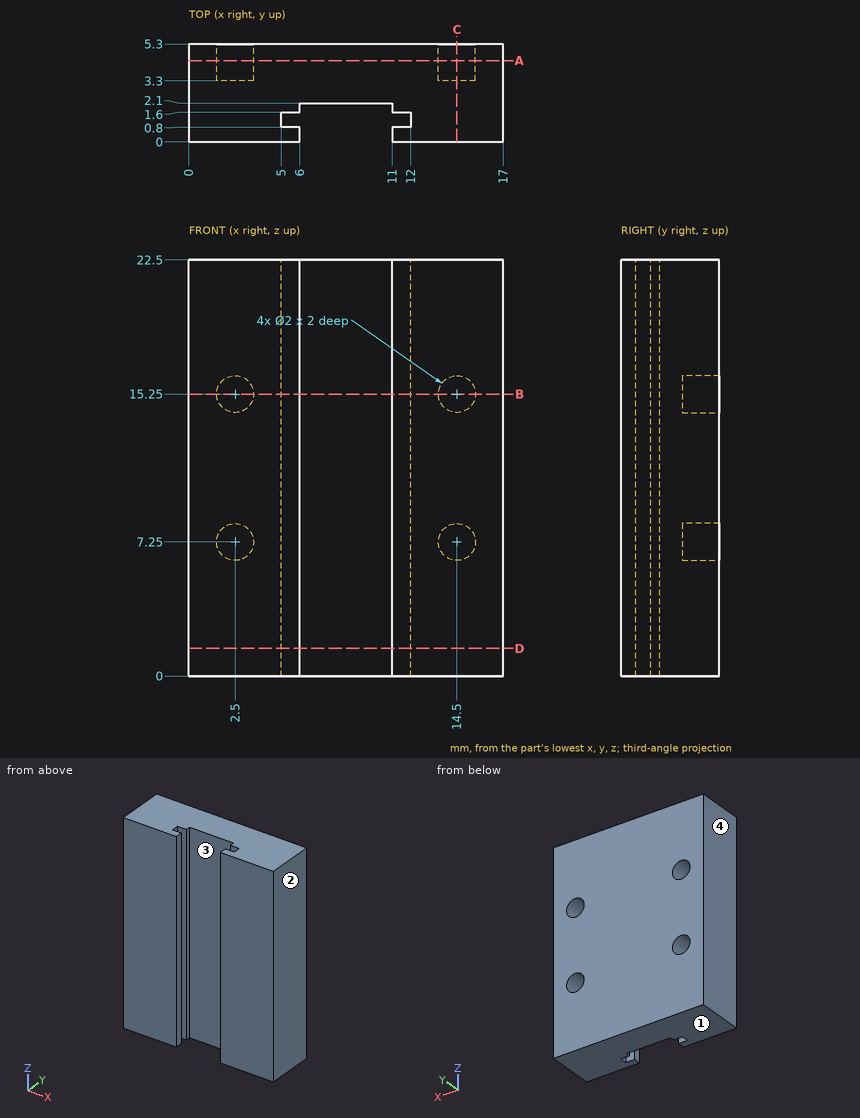
The drawing under review shows one solid part. Ordinate dimensions are in mm from its lowest x, y, z. Round coordinates to 2 decimals unless told otherwise and drop trailing zeros. Loops run counter-clockwise (first coordinate to the right, second up) from the corner with the lowest first, then second, coordinate; pieces in that order, holes last. Notation, with made-up numbers: (86.5, 12) -> (113.5, 12) arc R22 ccw to (113.5, 41) -> close; hole circle Ø4 at (66, 54.25). An arc over 180 degrees is marked (long way). Answer in a Markdown table with one row per item.
1) Consider section C-C, the plane x = 14.5. Write out the cut boundary in (y, z), plus the area to 3 significant figures.
Taken from the geometry:
| item | result |
|---|---|
| outline | (0, 0) -> (5.3, 0) -> (5.3, 6.25) -> (3.3, 6.25) -> (3.3, 8.25) -> (5.3, 8.25) -> (5.3, 14.25) -> (3.3, 14.25) -> (3.3, 16.25) -> (5.3, 16.25) -> (5.3, 22.5) -> (0, 22.5) -> close |
| area | 111 mm² |
2) Draft analysis for pull direction X (two halves, no side actions). For the marked faces 1, 2, 3 and 4, state which applies: pulls with the +X half, pulls with the -X half, needs draft (parallel to the pull), parting line crosses it, or undercut.
Taken from the geometry:
| item | result |
|---|---|
| face 1 | needs draft |
| face 2 | pulls with the +X half |
| face 3 | undercut |
| face 4 | pulls with the -X half |
3) Wall thickness on line 1 along X through (y, z) = (4.1, 7.25); line 2 along X through (y, z) = (1.55, 7.5); line 3 along Y through (x, z) = (9.75, 10.25): over which ranges is each line inside the solid? List them lowest first.
Taken from the geometry:
| item | result |
|---|---|
| line 1 | x = 0 to 1.5, 3.5 to 13.5, 15.5 to 17 |
| line 2 | x = 0 to 5, 12 to 17 |
| line 3 | y = 2.1 to 5.3 |
4) Consider section B-B, the plane z = 15.25. Write out the cut boundary in (x, y).
Taken from the geometry:
| item | result |
|---|---|
| outline | (0, 0) -> (6, 0) -> (6, 0.8) -> (5, 0.8) -> (5, 1.6) -> (6, 1.6) -> (6, 2.1) -> (11, 2.1) -> (11, 1.6) -> (12, 1.6) -> (12, 0.8) -> (11, 0.8) -> (11, 0) -> (17, 0) -> (17, 5.3) -> (15.5, 5.3) -> (15.5, 3.3) -> (13.5, 3.3) -> (13.5, 5.3) -> (3.5, 5.3) -> (3.5, 3.3) -> (1.5, 3.3) -> (1.5, 5.3) -> (0, 5.3) -> close |
5) For pin 1 Ø1.5 at (x, z) = (7.5, 8) entering from -Y; pin 2 Ø0.6 at (x, z) = (14, 15.5) entering from +Y, all flat-tipped, find the tip position at first contact; note any pin that passes through.
Taken from the geometry:
| item | result |
|---|---|
| pin 1 | stops at y = 2.1 |
| pin 2 | stops at y = 3.3 |
6) Consider section D-D, the plane z = 1.5. Write out the cut boundary in (x, y), plus the area to 3 significant figures.
Taken from the geometry:
| item | result |
|---|---|
| outline | (0, 0) -> (6, 0) -> (6, 0.8) -> (5, 0.8) -> (5, 1.6) -> (6, 1.6) -> (6, 2.1) -> (11, 2.1) -> (11, 1.6) -> (12, 1.6) -> (12, 0.8) -> (11, 0.8) -> (11, 0) -> (17, 0) -> (17, 5.3) -> (0, 5.3) -> close |
| area | 78.0 mm² |
7) Consider section A-A, the plane y = 4.4. Write out the cut boundary in (x, z), plus the area to 3 significant figures.
Taken from the geometry:
| item | result |
|---|---|
| outline | (0, 0) -> (17, 0) -> (17, 22.5) -> (0, 22.5) -> close; hole circle Ø2 at (2.5, 7.25); hole circle Ø2 at (2.5, 15.25); hole circle Ø2 at (14.5, 7.25); hole circle Ø2 at (14.5, 15.25) |
| area | 370 mm² |
